Autodesk Inventor part; units mm, degrees
ref_plane "YZ Plane" through (0, 0, 0) normal (1, 0, 0) x (0, 1, 0)
ref_plane "XZ Plane" through (0, 0, 0) normal (0, 1, 0) x (-1, 0, 0)
ref_plane "XY Plane" through (0, 0, 0) normal (0, 0, 1) x (1, 0, 0)
sketch "Sketch1" plane through (0, 0, 0) normal (0, 0, 1) x (1, 0, 0)
  line L0 (-11.9516, 53) -> (17.0484, 53)
  line L1 (23.0484, 47) -> (23.0484, 43)
  line L2 (3.0484, 23) -> (-1.9516, 23)
  line L3 (-11.9516, 33) -> (-11.9516, 53)
  arc A0 (23.0484, 47) -> (17.0484, 53) centre (17.0484, 47) ccw
  arc A1 (3.0484, 23) -> (23.0484, 43) centre (3.0484, 43) ccw
  arc A2 (-11.9516, 33) -> (-1.9516, 23) centre (-1.9516, 33) ccw
  point P0 (0, 0)
  point P1 (23.0484, 23)
  point P2 (-11.9516, 23)
  dimension "d0" = 6
  dimension "d1" = 30
  dimension "d2" = 35
  dimension "d3" = 20
  dimension "d4" = 10
extrude "Extrusion1" add sketch "Sketch1" along normal blind 7
sketch "Sketch2" plane through (0, 0, 7) normal (0, 0, 1) x (1, 0, 0)
  point P0 (0, 0)
  point P1 (2.9641, 39.4846)
hole "Hole1" at (2.9641, 39.4846, 7) direction (0, 0, -1) diameter 20 end through all
properties part number "McCrea_oko_walle"
The model under review builds one solid part; all positions refer to its coordinate system, in mm. Round coordinates to 2 decimals unless told otherwise and drop trailing zeros. Order: outer loops, then holes, each group sorted by start corner. A loop starts at its lowest first (then second) coordinate and runs counter-clockwise, first axis right, second up.
Item 1: For pin 1 (1.5 mm diameter, centred on y = 41.5, z = 3.5, fed in from +X); pin 2 (2 mm diameter, centred on x = 12, y = 38.5, fed in from +Z); pin 3 (1 mm diameter, centred on x = 14.5, z = 5.5, fed in from -Y), all flat-tipped, find the tip position at first contact; note any pin that passes through.
Working result:
pin 1: stops at x = 23.03
pin 2: stops at z = 7
pin 3: stops at y = 26.26
Item 2: Add section D-D, the plane x = 16. State the section outline as (y, z) points.
Working result:
outline: (27.76, 0) - (53, 0) - (53, 7) - (27.76, 7) - close
Item 3: Add section A-A, the plane y = 31.75. State the section outline as (x, z) points.
Working result:
outline: (-11.87, 0) - (-3.37, 0) - (-3.37, 7) - (-11.87, 7) - close; (9.3, 0) - (19.58, 0) - (19.58, 7) - (9.3, 7) - close
Item 4: To check wall thickness, follow probe 1 along Y at (x, z) = (6.5, 2); probe 2 along Y at (x, z) = (-1, 0.5); probe 3 along X at (y, z) = (47.5, 0.5). State the ranges of each line that lie inside material, in increasing order.
Working result:
probe 1: y = 23.3 to 30.13, 48.84 to 53
probe 2: y = 23 to 30.3, 48.67 to 53
probe 3: x = -11.95 to -3.02, 8.94 to 23.03
Item 5: Add section C-C, the plane z = 4.75. State the section outline as (x, y) points.
Working result:
outline: (-11.95, 33) arc R10 ccw to (-1.95, 23) - (3.05, 23) arc R20 ccw to (23.05, 43) - (23.05, 47) arc R6 ccw to (17.05, 53) - (-11.95, 53) - close; hole circle Ø20 at (2.96, 39.48)
Item 6: Add section B-B, the plane x = 5. State the section outline as (y, z) points.
Working result:
outline: (23.1, 0) - (29.69, 0) - (29.69, 7) - (23.1, 7) - close; (49.28, 0) - (53, 0) - (53, 7) - (49.28, 7) - close
Item 7: Draft analysis for pull direction X (two halves, no side actions). For faces 1 (the cylindrical face through (17.345, 29.014, 3.451)), 2 (the cylindrical face through (-0.04, 29.946, 3.451)), 3 (the flat face through (2, 53, 3)), 4 (the flat face through (-11.952, 43, 3)), state which applies: released by +X, released by -X, zero draft, split by the parting line, or undercut.
Working result:
face 1: released by +X
face 2: undercut
face 3: zero draft
face 4: released by -X
